Source: CAD feature listing. Evaluate the final solid. Frame: model axes, mm. Give positions to 0.01 mm unless a question says otherwise; leave off trailing zeros. Order: outer loops, then holes, each group sorted by start corner. A loop starts at its lowest first (then second) coordinate and runs counter-clockwise, first axis right, second up. Notation, with made-up numbers: M 41,-7.5 L 82,-7.5 A14 ccw 82,3.5 Z; hole C 76.25,35 d10. An arc over 180 degrees is marked long. Use CSV: the item, a comma, the result in double quotes. Start each with the question number.
1. Section query C-C, the plane z = 1.35. Return the cut outline in (x, y), plus the area to 3 significant figures.
2. Pin query (flat end, axial travel): P1, Ø1, axis at y = -42, z = 2, coming from the +X side. Return the tip coordinate at first contact, or that it passes through.
3. Section query B-B, the plane x = 15. Return the cut outline in (y, z).
4. Section query A-A, the plane y = -40. Return the cut outline in (x, z).
5. Line query: line 1 along Y through (x, z) = (40, 2.15); line 2 along Y through (x, z) = (15, 2.85); line 3 along X through (y, z) = (-33, 1.15). Output: solid intervals per line, ascending. Write a range as [from, to].
from build123d import *

# Parameters (mm, degrees)
SKETCH1_R           = 2.15
BOSS_EXTRUDE1_DEPTH = 4
FILLET1_R           = 2
CHAMFER1_SIZE       = 0.4


with BuildPart() as part:
    # Sketch1 → Boss-Extrude1 (new body)
    with BuildSketch(Plane.XY):
        Polygon((0, -50), (30, -50), (30, -30), (50, -30), (50, 0), (0, 0), align=None)
        with Locations((15, -40)):
            Circle(SKETCH1_R, mode=Mode.SUBTRACT)
        with Locations((40, -15)):
            Circle(SKETCH1_R, mode=Mode.SUBTRACT)
    extrude(amount=BOSS_EXTRUDE1_DEPTH)

    # Fillet1
    fillet1_edges = [part.edges().sort_by_distance(p)[0] for p in [
        (0, 0, 2),
        (50, 0, 2),
        (50, -30, 2),
        (30, -50, 2),
        (0, -50, 2),
    ]]
    fillet(fillet1_edges, radius=FILLET1_R)

    # Chamfer1
    chamfer1_edges = [part.edges().sort_by_distance(p)[0] for p in [
        (39, -30, 4),
        (12.85, -40, 0),
        (12.85, -40, 4),
        (37.85, -15, 0),
        (37.85, -15, 4),
        (0, -25, 0),
        (0, -25, 4),
        (25, 0, 0),
        (50, -15, 0),
        (30, -39, 0),
        (15, -50, 0),
        (29.414213562, -49.414213562, 0),
        (0.585786438, -49.414213562, 0),
        (49.414213562, -29.414213562, 0),
        (49.414213562, -0.585786438, 0),
        (0.585786438, -0.585786438, 0),
        (25, 0, 4),
        (15, -50, 4),
        (30, -39, 4),
        (50, -15, 4),
        (29.414213562, -49.414213562, 4),
        (0.585786438, -49.414213562, 4),
        (49.414213562, -29.414213562, 4),
        (49.414213562, -0.585786438, 4),
        (0.585786438, -0.585786438, 4),
        (39, -30, 0),
    ]]
    chamfer(chamfer1_edges, length=CHAMFER1_SIZE)


solid = part.part
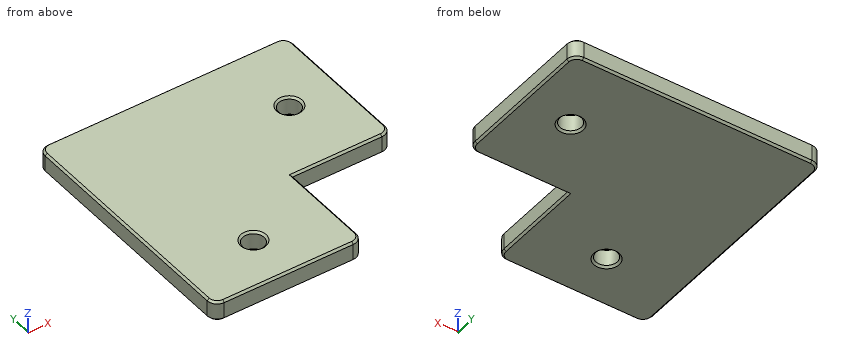
Result set:
1,outline,"M 0,-48 A2 ccw 2,-50 L 28,-50 A2 ccw 30,-48 L 30,-30 L 48,-30 A2 ccw 50,-28 L 50,-2 A2 ccw 48,0 L 2,0 A2 ccw 0,-2 Z; hole C 15,-40 d4.3; hole C 40,-15 d4.3"
1,area,"2,070 mm2"
2,P1,"x = 30"
3,outline,"M -50,0.4 L -49.6,0 L -42.55,0 L -42.15,0.4 L -42.15,3.6 L -42.55,4 L -49.6,4 L -50,3.6 Z; M -37.85,0.4 L -37.45,0 L -0.4,0 L 0,0.4 L 0,3.6 L -0.4,4 L -37.45,4 L -37.85,3.6 Z"
4,outline,"M 0,0.4 L 0.4,0 L 12.45,0 L 12.85,0.4 L 12.85,3.6 L 12.45,4 L 0.4,4 L 0,3.6 Z; M 17.15,0.4 L 17.55,0 L 29.6,0 L 30,0.4 L 30,3.6 L 29.6,4 L 17.55,4 L 17.15,3.6 Z"
5,line 1,"[-30, -17.15], [-12.85, 0]"
5,line 2,"[-50, -42.15], [-37.85, 0]"
5,line 3,"[0, 30]"
